Input: part model. Units: mm. Frame: model coordinates. A direction names the side the tool comes from. Coordinates: 2 decimals unless noted, no trailing zeros. Write each loop counter-clockwise with the first axis right and the second up, starting at its lowest first coordinate (ties: lowest second). Pieces come first, ordered by that corner, then holes. Notation, with made-up numbers: (61.25, 68) - (85.25, 68) arc R30 ccw to (85.25, 96) - close; hole circle Ø11 at (72, 40). An arc over 180 degrees is marked (long way). One line per question, with ' | ' between items. Start each with the question number.
1) Section query D-D on y = -52.5. Return loops of the section in (x, z), and give its area (3 significant figures).
2) First-contact query: P1, Ø1, axis at x = 62.5, y = -9, coming from the +Z side; P2, Ø3, axis at x = -13.5, z = -28.5, coming from the -Y side; P3, Ø1.5, axis at x = 104, y = -19, coming from the +Z side; P4, Ø14.5, axis at x = 33.5, z = -18.5, coming from the +Y side. Flat tips, straight axial feed; report the tip coordinate or a pass-through.
3) Line query: line 1 (Z direction, x = 27.5, y = -27.5); line 2 (X direction, y = 0.5, z = 23); line 3 (Z direction, x = -45.5, y = -15.5). Output: solid intervals per line, ascending.
4) Section query B-B on x = -51.5. Return loops of the section in (y, z), and give its area (3 significant figures).
5) Draft query along Z for faces 5 (the flat face through (105.411, 7.481, 25.771)), 6 (the flat face through (-95, -4, 1)), 7 (the cylindrical face through (-16.01, -19.16, -64.15)), 8 (the flat face through (56.499, 7.481, -41.664)). Return one class per face: released by +Z, released by -Z, zero draft, split by the parting line, or undercut.
6) Reachability of faces 1 (the flat face through (33.66, -14.44, 23.31)), 2 (the cylindrical face through (-78.99, -3.94, 64.15)), 3 (the flat face through (100, -42, -67)), 4 (the cylindrical face through (149, -43, -52)) from +Z, -Z, +X, -X, +Y, -Y: full face, straight path, thin tool, end or side. Return the list, or none.
7) Section query C-C on x = 70. Return loops of the section in (y, z), and give its area (3 significant figures).
```python
from build123d import *

# Parameters (mm, degrees)
BOSS_EXTRUDE1_DEPTH = 80
CUT_EXTRUDE1_REACH  = 42
CUT_EXTRUDE2_REACH  = 247
SKETCH3_W           = 134
SKETCH3_H           = 8.658823529
SKETCH4_R           = 25
SKETCH4_R_2         = 20
BOSS_EXTRUDE2_DEPTH = 30
SKETCH5_W           = 50
SKETCH5_H           = 30
BOSS_EXTRUDE4_DEPTH = 5
FILLET1_R           = 5
CUT_EXTRUDE5_REACH  = 47
SKETCH11_R          = 37.5
SKETCH11_R_2        = 30
BOSS_EXTRUDE6_DEPTH = 50
SKETCH12_R          = 55
SKETCH12_R_2        = 50
BOSS_EXTRUDE7_DEPTH = 40
RIB1_REACH          = 82
SKETCH13_WALL_W     = 175.462912018
SKETCH13_WALL_H     = 5
CIRPATTERN1_COUNT   = 10


with BuildPart() as part:
    # Sketch1 → Boss-Extrude1 (new body, symmetric)
    with BuildSketch(Plane.XY):
        Polygon((150, -40), (150, -35), (0, -35), (0, 0), (-95, 0), (-95, -8), (-10, -40), align=None)
    extrude(amount=BOSS_EXTRUDE1_DEPTH, both=True)

    # Cut-Extrude1: up to this plane
    cut_extrude1_end = Plane(origin=(-95, -8, 80), z_dir=(0.352329759, 0.935875922, 0))
    # Sketch2 → Cut-Extrude1 (cut, up to the surface)
    with BuildSketch(Plane(origin=(0, 0, 0), x_dir=(-1, 0, 0), z_dir=(0, 1, 0)), mode=Mode.PRIVATE) as cut_extrude1_sk1:
        with BuildLine():
            Line((23, 67), (72, 67))
            ThreePointArc((72, 67), (79.071067812, 64.071067812), (82, 57))
            Line((82, 57), (82, -57))
            ThreePointArc((82, -57), (79.071067812, -64.071067812), (72, -67))
            Line((72, -67), (23, -67))
            ThreePointArc((23, -67), (15.928932188, -64.071067812), (13, -57))
            Line((13, -57), (13, 57))
            ThreePointArc((13, 57), (15.928932188, 64.071067812), (23, 67))
        make_face()
    cut_extrude1_tool1 = split(extrude(cut_extrude1_sk1.sketch, amount=-CUT_EXTRUDE1_REACH, mode=Mode.PRIVATE), bisect_by=cut_extrude1_end, keep=Keep.BOTH, mode=Mode.PRIVATE)
    add(cut_extrude1_tool1.solids().sort_by_distance((-47.5, 0, 0))[0], mode=Mode.SUBTRACT)

    # Sketch3 → Cut-Extrude2 (cut, up to next)
    with BuildSketch(Plane.ZY.offset(95), mode=Mode.PRIVATE) as cut_extrude2_sk1:
        with Locations((0, -12.329411764)):
            Rectangle(SKETCH3_W, SKETCH3_H)
    cut_extrude2_tool1 = extrude(cut_extrude2_sk1.sketch, amount=-CUT_EXTRUDE2_REACH, mode=Mode.PRIVATE) & part.part
    add(cut_extrude2_tool1.solids().sort_by_distance((-95, -12.329412, 0))[0], mode=Mode.SUBTRACT)

    # Sketch4 → Boss-Extrude2 (add)
    with BuildSketch(Plane(origin=(0, -40, 0), x_dir=(-1, 0, 0), z_dir=(0, -1, 0))):
        with Locations((-70, 0)):
            Circle(SKETCH4_R)
        with Locations(Location((-70, 0, 0), (0, 0, 180))):  # turned: the seam where the file's is
            Circle(SKETCH4_R_2, mode=Mode.SUBTRACT)
    extrude(amount=BOSS_EXTRUDE2_DEPTH)

    # Sketch5 → Boss-Extrude4 (add)
    with BuildSketch(Plane(origin=(0, -40, 0), x_dir=(-1, 0, 0), z_dir=(0, -1, 0))):
        with Locations((-125, 65)):
            Rectangle(SKETCH5_W, SKETCH5_H)
        with Locations((-15, 65)):
            Rectangle(SKETCH5_W, SKETCH5_H)
        with Locations((-15, -65)):
            Rectangle(SKETCH5_W, SKETCH5_H)
        with Locations((-125, -65)):
            Rectangle(SKETCH5_W, SKETCH5_H)
    extrude(amount=BOSS_EXTRUDE4_DEPTH)

    # Fillet1
    fillet1_edges = [part.edges().sort_by_distance(p)[0] for p in [
        (150, -42.5, 50),
        (100, -42.5, 50),
        (150, -42.5, -50),
        (100, -42.5, -50),
        (40, -42.5, -50),
        (40, -42.5, 50),
    ]]
    fillet(fillet1_edges, radius=FILLET1_R)

    # Sketch10 → Cut-Extrude5 (cut, up to next)
    with BuildSketch(Plane(origin=(0, -45, 0), x_dir=(-1, 0, 0), z_dir=(0, -1, 0)), mode=Mode.PRIVATE) as cut_extrude5_sk1:
        with BuildLine():
            Line((-130, 69), (-115, 69))
            ThreePointArc((-115, 69), (-111, 65), (-115, 61))
            Line((-115, 61), (-130, 61))
            ThreePointArc((-130, 61), (-134, 65), (-130, 69))
        make_face()
    cut_extrude5_tool1 = extrude(cut_extrude5_sk1.sketch, amount=-CUT_EXTRUDE5_REACH, mode=Mode.PRIVATE) & part.part
    add(cut_extrude5_tool1.solids().sort_by_distance((122.5, -45, -65))[0], mode=Mode.SUBTRACT)
    # Sketch10 → Cut-Extrude5 (cut, up to next)
    with BuildSketch(Plane(origin=(0, -45, 0), x_dir=(-1, 0, 0), z_dir=(0, -1, 0)), mode=Mode.PRIVATE) as cut_extrude5_sk2:
        with BuildLine():
            Line((-10, 69), (-25, 69))
            ThreePointArc((-25, 69), (-29, 65), (-25, 61))
            Line((-25, 61), (-10, 61))
            ThreePointArc((-10, 61), (-6, 65), (-10, 69))
        make_face()
    cut_extrude5_tool2 = extrude(cut_extrude5_sk2.sketch, amount=-CUT_EXTRUDE5_REACH, mode=Mode.PRIVATE) & part.part
    add(cut_extrude5_tool2.solids().sort_by_distance((17.5, -45, -65))[0], mode=Mode.SUBTRACT)
    # Sketch10 → Cut-Extrude5 (cut, up to next)
    with BuildSketch(Plane(origin=(0, -45, 0), x_dir=(-1, 0, 0), z_dir=(0, -1, 0)), mode=Mode.PRIVATE) as cut_extrude5_sk3:
        with BuildLine():
            Line((-130, -69), (-115, -69))
            ThreePointArc((-115, -69), (-111, -65), (-115, -61))
            Line((-115, -61), (-130, -61))
            ThreePointArc((-130, -61), (-134, -65), (-130, -69))
        make_face()
    cut_extrude5_tool3 = extrude(cut_extrude5_sk3.sketch, amount=-CUT_EXTRUDE5_REACH, mode=Mode.PRIVATE) & part.part
    add(cut_extrude5_tool3.solids().sort_by_distance((122.5, -45, 65))[0], mode=Mode.SUBTRACT)
    # Sketch10 → Cut-Extrude5 (cut, up to next)
    with BuildSketch(Plane(origin=(0, -45, 0), x_dir=(-1, 0, 0), z_dir=(0, -1, 0)), mode=Mode.PRIVATE) as cut_extrude5_sk4:
        with BuildLine():
            Line((-10, -69), (-25, -69))
            ThreePointArc((-25, -69), (-29, -65), (-25, -61))
            Line((-25, -61), (-10, -61))
            ThreePointArc((-10, -61), (-6, -65), (-10, -69))
        make_face()
    cut_extrude5_tool4 = extrude(cut_extrude5_sk4.sketch, amount=-CUT_EXTRUDE5_REACH, mode=Mode.PRIVATE) & part.part
    add(cut_extrude5_tool4.solids().sort_by_distance((17.5, -45, 65))[0], mode=Mode.SUBTRACT)

    # Sketch11 → Boss-Extrude6 (add)
    with BuildSketch(Plane(origin=(0, -35, 0), x_dir=(-1, 0, 0), z_dir=(0, 1, 0))):
        with Locations(Location((-70, 0, 0), (0, 0, 180))):  # turned: the seam where the file's is
            Circle(SKETCH11_R)
        with Locations(Location((-70, 0, 0), (0, 0, 90))):  # turned: the seam where the file's is
            Circle(SKETCH11_R_2, mode=Mode.SUBTRACT)
    extrude(amount=BOSS_EXTRUDE6_DEPTH)

    # Sketch12 → Boss-Extrude7 (add)
    with BuildSketch(Plane(origin=(0, -35, 0), x_dir=(-1, 0, 0), z_dir=(0, 1, 0))):
        with Locations(Location((-70, 0, 0), (0, 0, 180))):  # turned: the seam where the file's is
            Circle(SKETCH12_R)
        with Locations(Location((-70, 0, 0), (0, 0, 90))):  # turned: the seam where the file's is
            Circle(SKETCH12_R_2, mode=Mode.SUBTRACT)
    extrude(amount=BOSS_EXTRUDE7_DEPTH)

    # Sketch13 wall → Rib1 (add, up to next)
    with BuildSketch(Plane(origin=(26.25, 7.5, 0), x_dir=(0.928476691, 0.371390676, 0), z_dir=(-0.371390676, 0.928476691, 0)), mode=Mode.PRIVATE) as rib1_sk1:
        Rectangle(SKETCH13_WALL_W, SKETCH13_WALL_H)
    rib1_tool1 = extrude(rib1_sk1.sketch, amount=-RIB1_REACH, mode=Mode.PRIVATE) - part.part
    rib1 = rib1_tool1.solids().sort_by_distance((26.25, 7.5, 0))[0]
    add(rib1)

    # CirPattern1: Rib1 ×10 about axis
    cirpattern1_axis = Axis((70, 0, 0), (0, 1, 0))
    for i in range(1, CIRPATTERN1_COUNT):
        add(rib1.rotate(cirpattern1_axis, i * 360 / CIRPATTERN1_COUNT))


solid = part.part
```
Answer key:
1) outline: circle Ø50 at (70, 0); hole circle Ø40 at (70, 0) | area: 707 mm²
2) P1: z = 54.55 | P2: y = -39.25 | P3: z = 43.81 | P4: y = 15
3) line 1: -34.91 to -26.34, -2.5 to 2.5, 26.34 to 34.91 | line 2: 20.04 to 25.6, 34.09 to 50.74, 89.26 to 105.91, 114.4 to 119.96 | line 3: -80 to -67, 67 to 80
4) outline: (-24.38, -80) - (0, -80) - (0, -67) - (-24.38, -67) - close; (-24.38, 67) - (0, 67) - (0, 80) - (-24.38, 80) - close | area: 634 mm²
5) face 5: released by +Z | face 6: zero draft | face 7: undercut | face 8: released by -Z
6) face 1: +Y | face 2: +Y, -Y | face 3: +Z, -Z, -Y | face 4: +X, -Y
7) outline: (-70, -25) - (-40, -25) - (-40, -80) - (-35, -80) - (-35, -55) - (5, -55) - (5, -50) - (-35, -50) - (-35, -37.5) - (15, -37.5) - (15, -30) - (-35, -30) - (-35, 30) - (15, 30) - (15, 37.5) - (-35, 37.5) - (-35, 50) - (5, 50) - (5, 55) - (-35, 55) - (-35, 80) - (-40, 80) - (-40, 25) - (-70, 25) - (-70, 20) - (-40, 20) - (-40, -20) - (-70, -20) - close | area: 2,250 mm²
